from build123d import *

# Parameters (mm, degrees)
HEX_2_DEPTH                = 6.096
SKETCH2_R                  = 7.9375
SKETCH2_R_2                = 3.2639
ROTARY_SHAFT_DEPTH         = 15.621
SKETCH3_R                  = 2.2225
SHAFT_SETSCREW_HOLES_DEPTH = 20.235993697
SKETCH4_R                  = 2.2225
CUT_EXTRUDE2_DEPTH         = 20.235993861


with BuildPart() as part:
    # Sketch1 → Hex 2 (new body)
    with BuildSketch(Plane(origin=(0, 0, 0), x_dir=(0, 0, -1), z_dir=(1, 0, 0))):
        Polygon((-3.534191938, 6.1214), (3.534191938, 6.1214), (7.068383876, 0), (3.534191938, -6.1214), (-3.534191938, -6.1214), (-7.068383876, 0), align=None)
    extrude(amount=HEX_2_DEPTH)

    # Sketch2 → Rotary_Shaft (add)
    with BuildSketch(Plane.ZY):
        with Locations(Location((0, 0, 0), (0, 0, 180))):
            Circle(SKETCH2_R)
        with Locations(Location((0, 0, 0), (0, 0, 180))):
            Circle(SKETCH2_R_2, mode=Mode.SUBTRACT)
    extrude(amount=ROTARY_SHAFT_DEPTH)

    # Sketch3 → Shaft-SetScrew-Holes (cut, through all)
    with BuildSketch(Plane(origin=(0, 0, 0), x_dir=(1, 0, 0), z_dir=(0, 1, 0))):
        with Locations(Location((-11.43, 0, 0), (0, 0, 90))):
            Circle(SKETCH3_R)
        with Locations(Location((-3.81, 0, 0), (0, 0, 90))):
            Circle(SKETCH3_R)
    extrude(amount=SHAFT_SETSCREW_HOLES_DEPTH, mode=Mode.SUBTRACT)

    # Sketch4 → Cut-Extrude2 (cut, through all)
    with BuildSketch(Plane.ZY):
        Circle(SKETCH4_R)
    extrude(amount=-CUT_EXTRUDE2_DEPTH, mode=Mode.SUBTRACT)


solid = part.part
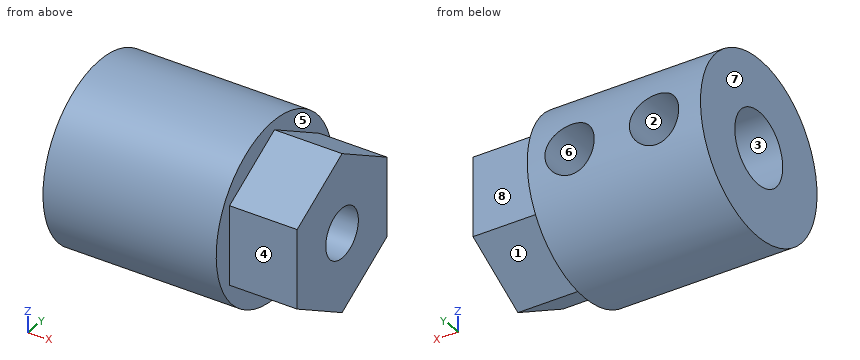
The listing builds one solid part. Answer for the finished solid, in the listing's coordinates (mm). Face numbers are marked on the shaded views. A direction names the side the tool comes from. Give positions to 0.01 mm unless a question says otherwise; leave off trailing zeros. Loops run counter-clockwise (first coordinate to the right, second up) from the corner with the lowest first, then second, coordinate; pieces in that order, holes last.
Item 1: A tool of negligible diameter and unlimited length cuts with its end or side. For the marked faces 1, 2, 3, 4 and 5, from which of +Z, -Z, +X, -X, +Y, -Y can it reach the whole face along a straight path? Write none if from no direction.
Derived:
face 1: -Z, +X, +Y
face 2: +Y
face 3: -X
face 4: +Z, -Z, +X, -Y
face 5: +X
Item 2: Each of these flat-tipped pins is pushed along its axis until it touches: pin 1 Ø1.5 at (x, y) = (-13, -2) entering from +Z; pin 2 Ø3.5 at (x, z) = (-11.43, 0) entering from +Y; pin 3 Ø3 at (x, z) = (3, -1) entering from -Y; pin 4 Ø3.5 at (y, z) = (0, 0) entering from +X. Where does it stop, or does it pass through?
Derived:
pin 1: stops at z = 7.84
pin 2: stops at y = -2.76
pin 3: stops at y = -6.12
pin 4: passes through
Item 3: A cutting plane is placed at C-C (y = 5.75). Give the vertices of the cut face in (x, z) (1 decimal).
Derived:
outline: (-15.6, -5.5) - (0, -5.5) - (0, -3.7) - (6.1, -3.7) - (6.1, 3.7) - (0, 3.7) - (0, 5.5) - (-15.6, 5.5) - close; hole circle Ø4.4 at (-11.4, 0); hole circle Ø4.4 at (-3.8, 0)
Item 4: Find the intervals of material crossed by line 1 along X through (y, z) = (6.3, 0); line 2 along X through (y, z) = (3.75, 0); line 3 along Y through (x, z) = (3.5, 0), in increasing order.
Derived:
line 1: x = -15.62 to -13.65, -9.21 to -6.03, -1.59 to 0
line 2: x = -15.62 to -13.65, -9.21 to -6.03, -1.59 to 6.1
line 3: y = -6.12 to -2.22, 2.22 to 6.12
Item 5: Determine the mould class of the marked faces 6, 7 and 8 for opening direction X: +X half, -X half, draft (parallel to the pull), parting line (faces both ways), or undercut.
Derived:
face 6: undercut
face 7: -X half
face 8: draft
Item 6: A cutting plane is placed at A-A (z = -1). Give the vertices of the cut face in (x, y).
Derived:
outline: (-15.62, -7.87) - (0, -7.87) - (0, -6.12) - (6.1, -6.12) - (6.1, -1.98) - (0, -1.98) - (0, -3.11) - (-15.62, -3.11) - close; (-15.62, 3.11) - (-13.41, 3.11) - (-13.41, 7.87) - (-15.62, 7.87) - close; (-9.45, 3.11) - (-5.79, 3.11) - (-5.79, 7.87) - (-9.45, 7.87) - close; (-1.83, 3.11) - (0, 3.11) - (0, 1.98) - (6.1, 1.98) - (6.1, 6.12) - (0, 6.12) - (0, 7.87) - (-1.83, 7.87) - close
Item 7: A cutting plane is placed at D-D (y = -4). Give the vertices of the cut face in (x, z), then the cut area to 3 significant figures.
Derived:
outline: (-15.62, -6.86) - (0, -6.86) - (0, -4.76) - (6.1, -4.76) - (6.1, 4.76) - (0, 4.76) - (0, 6.86) - (-15.62, 6.86) - close
area: 272 mm2
Item 8: A cutting plane is placed at B-B (x = 3). Give the vertices of the cut face in (y, z) (1 decimal), then the cut area to 3 significant figures.
Derived:
outline: (-6.1, -3.5) - (0, -7.1) - (6.1, -3.5) - (6.1, 3.5) - (0, 7.1) - (-6.1, 3.5) - close; hole circle Ø4.4 at (0, 0)
area: 114 mm2
